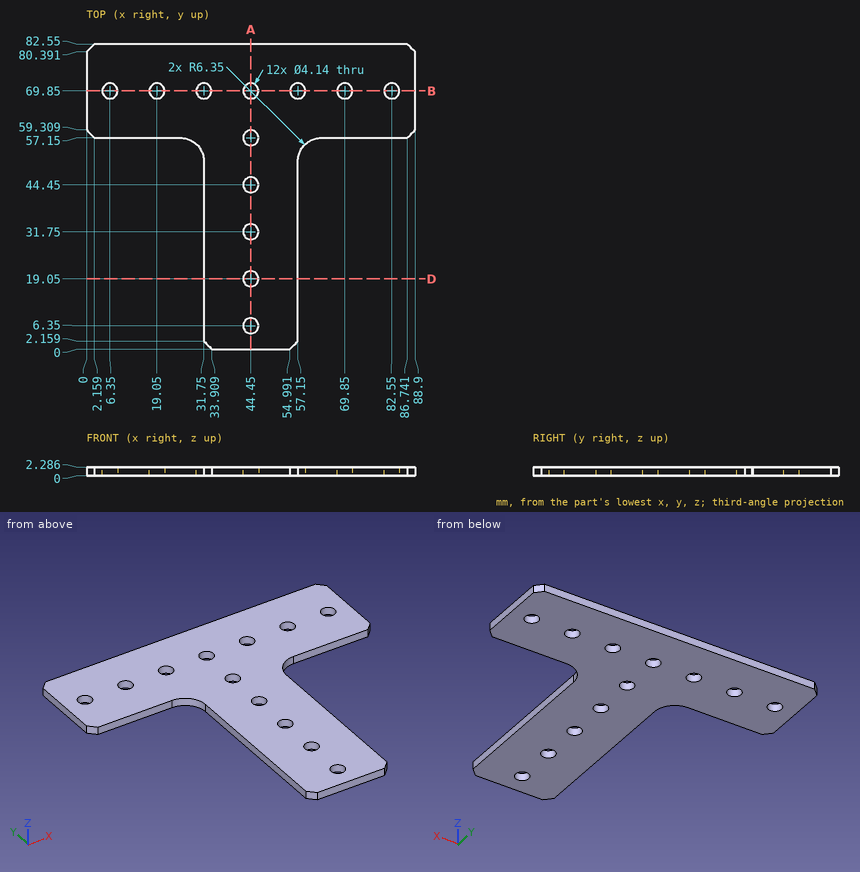
Study the drawing (mm; zero at the part's minimum x, y, z) and answer. Round coordinates to 2 decimals unless told otherwise and drop trailing zeros. Loops run counter-clockwise (first coordinate to the right, second up) from the corner with the lowest first, then second, coordinate; pieces in that order, holes last. Notation, with made-up numbers: (15.5, 3) -> (36.5, 3) arc R17 ccw to (36.5, 19) -> close; hole circle Ø11 at (-36, -39). An arc over 180 degrees is marked (long way). Use one line per item in the form item = value.
1. Find the intervals of material crossed by probe 1 along X at (y, z) = (44.5, 1.4); probe 2 along Y at (x, z) = (19.05, 1.05); probe 3 along Y at (x, z) = (63.5, 1.2), in increasing order. Write a range as [from, to].
Answer key:
probe_1 = [31.75, 42.38], [46.52, 57.15]
probe_2 = [57.15, 67.78], [71.92, 82.55]
probe_3 = [57.15, 82.55]
2. Flat-ended cylindrical pins translate along their axes: pin 1 Ø0.7 at (x, z) = (79.5, 1.5) entering from -Y; pin 2 Ø0.7 at (y, z) = (19, 1) entering from +X. Find the tip coordinate at first contact, or state that the pin passes through.
Answer key:
pin_1 = 57.15
pin_2 = 57.15
3. The part is cut by section D-D on y = 19.05. Determine the outline of the cut face in (x, z).
Answer key:
outline = (31.75, 0) -> (42.38, 0) -> (42.38, 2.29) -> (31.75, 2.29) -> close; (46.52, 0) -> (57.15, 0) -> (57.15, 2.29) -> (46.52, 2.29) -> close
4. The part is cut by section A-A on x = 44.45. Determine the outline of the cut face in (y, z), and give its area (3 significant figures).
Answer key:
outline = (0, 0) -> (4.28, 0) -> (4.28, 2.29) -> (0, 2.29) -> close; (8.42, 0) -> (16.98, 0) -> (16.98, 2.29) -> (8.42, 2.29) -> close; (21.12, 0) -> (29.68, 0) -> (29.68, 2.29) -> (21.12, 2.29) -> close; (33.82, 0) -> (42.38, 0) -> (42.38, 2.29) -> (33.82, 2.29) -> close; (46.52, 0) -> (55.08, 0) -> (55.08, 2.29) -> (46.52, 2.29) -> close; (59.22, 0) -> (67.78, 0) -> (67.78, 2.29) -> (59.22, 2.29) -> close; (71.92, 0) -> (82.55, 0) -> (82.55, 2.29) -> (71.92, 2.29) -> close
area = 132 mm²
5. The part is cut by section B-B on y = 69.85. Give the number of separate pieces and of enclosed holes in the cut face, and give its area (3 significant figures).
Answer key:
separate_pieces = 8
enclosed_holes = 0
area = 137 mm²
